The model under review builds one solid part; all positions refer to its coordinate system, in mm. Round coordinates to 2 decimals unless told otherwise and drop trailing zeros. Order: outer loops, then holes, each group sorted by start corner. A loop starts at its lowest first (then second) coordinate and runs counter-clockwise, first axis right, second up. Notation, with made-up numbers: (11, 15.25) -> (49, 15.25) arc R20 ccw to (49, 23.25) -> close; hole circle Ø5 at (56.25, 50). An arc over 180 degrees is marked (long way). Use a Markdown table: item, result. Add a question column.
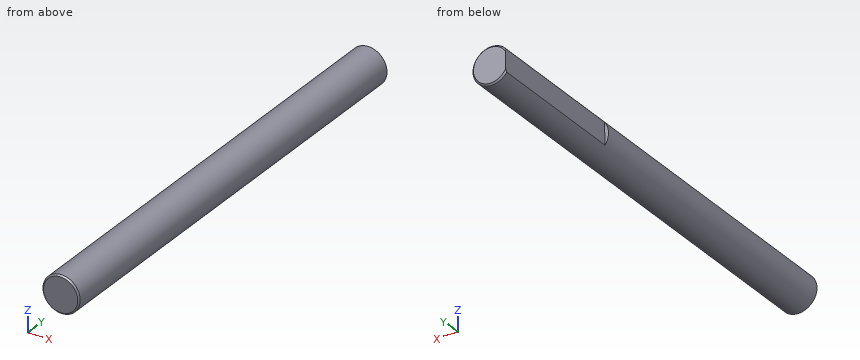
```python
from build123d import *

# Parameters (mm, degrees)
SKETCH1_R               = 2.5
BOSS_EXTRUDE1_DEPTH     = 62.2
CUT_EXTRUDE1_DEPTH      = 63.300401283
CUT_EXTRUDE1_DEPTH_BACK = 20
CHAMFER1_SIZE           = 0.2
CHAMFER2_SIZE           = 0.2


with BuildPart() as part:
    # Sketch1 → Boss-Extrude1 (new body)
    with BuildSketch(Plane(origin=(0, 0, 0), x_dir=(1, 0, 0), z_dir=(0, 1, 0))):
        with Locations(Location((0, 0, 0), (0, 0, 90))):
            Circle(SKETCH1_R)
    extrude(amount=BOSS_EXTRUDE1_DEPTH)

    # Sketch2 → Cut-Extrude1 (cut, two sides: drawn at the far end of the back side and taken through both)
    with BuildSketch(Plane(origin=(0, 62.2, 0), x_dir=(1, 0, 0), z_dir=(0, 1, 0)).offset(-CUT_EXTRUDE1_DEPTH_BACK)):
        with BuildLine():
            Line((-2.039291674, 1.446129132), (-1.959285636, -1.55280385))
            ThreePointArc((-1.959285636, -1.55280385), (-2.499110819, -0.066671699), (-2.039291674, 1.446129132))
        make_face()
    extrude(amount=CUT_EXTRUDE1_DEPTH + CUT_EXTRUDE1_DEPTH_BACK, mode=Mode.SUBTRACT)

    # Chamfer1
    chamfer1_edges = [part.edges().sort_by_distance(p)[0] for p in [
        (2.250778713, 62.2, 1.088115429),
    ]]
    chamfer(chamfer1_edges, length=CHAMFER1_SIZE)

    # Chamfer2
    chamfer2_edges = [part.edges().sort_by_distance(p)[0] for p in [
        (0, 0, 2.5),
    ]]
    chamfer(chamfer2_edges, length=CHAMFER2_SIZE)


solid = part.part
```
Q1. Add section B-B, the plane y = 17. Give the boundary of the cut face in (x, z), then the cut area to 3 significant figures.
Q2. To check wall thickness, follow line 1 along Z through (x, y) = (0.1, 46.5); line 2 along X through (y, z) = (25.5, -1.55); line 3 along Z through (x, y) = (2, 21). State the ranges of each line that lie inside material, in increasing order.
Q3. For pin 1 (2 mm diameter, centred on y = 22.5, z = 2, fed in from +X), flat-tipped, find the tip position at first contact; note if it passes through.
Q4. Add section A-A, the plane z = 0. Give the boundary of the cut face in (x, y), then the cut area to 3 significant figures.
Return value:
| question | item | result |
|---|---|---|
| 1 | outline | circle Ø5 at (0, 0) |
| 1 | area | 19.6 mm² |
| 2 | line 1 | -2.5 to 2.5 |
| 2 | line 2 | -1.96 to 1.96 |
| 2 | line 3 | -1.5 to 1.5 |
| 3 | pin 1 | x = 2.29 |
| 4 | outline | (-2.5, 0.2) -> (-2.3, 0) -> (2.3, 0) -> (2.5, 0.2) -> (2.5, 62) -> (2.3, 62.2) -> (-2, 62.2) -> (-2, 42.2) -> (-2.5, 42.2) -> close |
| 4 | area | 301 mm² |
